Input: part model. Units: mm. Frame: model coordinates. Face numbers are marked on the shaded views. A direction names the side the tool comes from. Give positions to 0.01 mm unless a question says otherwise; leave off trailing zeros. Write each loop counter-clockwise with the first axis right and the second up, starting at its lowest first coordinate (ties: lowest second). Pieces come first, ordered by that corner, then holes.
```python
from build123d import *

# Parameters (mm, degrees)
F0_W     = 200
F0_H     = 50
F1_DEPTH = 40
F2_W     = 38
F2_H     = 28
F3_DEPTH = 200.001
F4_R     = 1
F5_DEPTH = 8
F6_R     = 1
F7_DEPTH = 8


with BuildPart() as f1:
    # F0 (on Top) → F1 (new body)
    with BuildSketch(Plane.XY):
        with Locations((40.836534, -29.115389)):
            Rectangle(F0_W, F0_H)
    extrude(amount=F1_DEPTH)

    # F2 (on face) → F3 (cut, through all)
    with BuildSketch(Plane(origin=(-59.163466, 0, 0), x_dir=(0, -1, 0), z_dir=(-1, 0, 0))):
        with Locations((29.115389, 20)):
            Rectangle(F2_W, F2_H)
    extrude(amount=-F3_DEPTH, mode=Mode.SUBTRACT)

    # F4 (on face) → F5 (cut)
    with BuildSketch(Plane(origin=(-59.163466, 0, 0), x_dir=(0, -1, 0), z_dir=(-1, 0, 0))):
        with Locations((8.115389, 36)):
            Circle(F4_R)
        with Locations((8.115389, 4)):
            Circle(F4_R)
        with Locations((50.115389, 4)):
            Circle(F4_R)
        with Locations((50.115389, 36)):
            Circle(F4_R)
    extrude(amount=-F5_DEPTH, mode=Mode.SUBTRACT)

    # F6 (on face) → F7 (cut)
    with BuildSketch(Plane.YZ.offset(140.836534)):
        with Locations((-50.115389, 36)):
            Circle(F6_R)
        with Locations((-8.115389, 36)):
            Circle(F6_R)
        with Locations((-8.115389, 4)):
            Circle(F6_R)
        with Locations((-50.115389, 4)):
            Circle(F6_R)
    extrude(amount=-F7_DEPTH, mode=Mode.SUBTRACT)


solid = f1.part
```
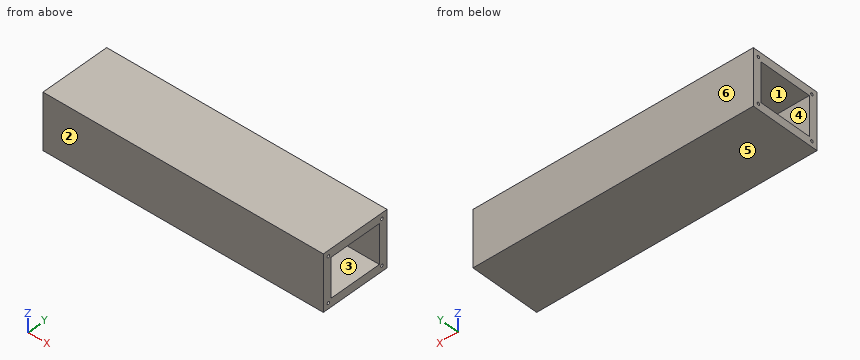
Item 1: Mould query, pull axis Y, two halves, no side actions, for the marked faces 3, 4, 5 and 6. Classes: +Y half, -Y half, draft (parallel to the pull), parting line (faces both ways), or undercut.
Item 2: Set-up query: the marked faces 1 and 2. Return all of +Z, -Z, +X, -X, +Y, -Y with unobstructed straight access to the full face (end or side cutting, diameter ignored); none if empty.
Item 3: Section C-C (y = -14). Return loops of the section in (x, z), and give its area (3 significant figures).
Item 4: Ray query, line 1 (Y direction, x = 104.5, z = 30.5); line 2 (Z direction, x = -46.5, y = -14.5). Return the intervals inside material, ascending.
Item 5: Section B-B (z = 10.5). Return loops of the section in (x, y).
Item 6: Section A-A (x = 84). Return loops of the section in (y, z), and give its area (3 significant figures).
Item 7: Pin query (flat end, axial travel): pin 1 (1 mm diameter, centred on x = 27.5, y = -41, fed in from -Z); pin 2 (0.6 mm diameter, centred on y = -49.5, z = 4, fed in from +X); pin 3 (1.8 mm diameter, centred on y = -8.12, z = 36, fed in from -X). Return the tip coordinate at first contact, or that it passes through.
Solved:
1. face 3: undercut
1. face 4: undercut
1. face 5: draft
1. face 6: +Y half
2. face 1: +X, -X
2. face 2: +Z, -Z, +X, -X, -Y
3. outline: (-59.16, 0) - (140.84, 0) - (140.84, 6) - (-59.16, 6) - close; (-59.16, 34) - (140.84, 34) - (140.84, 40) - (-59.16, 40) - close
3. area: 2,400 mm2
4. line 1: y = -54.12 to -48.12, -10.12 to -4.12
4. line 2: z = 0 to 6, 34 to 40
5. outline: (-59.16, -54.12) - (140.84, -54.12) - (140.84, -48.12) - (-59.16, -48.12) - close; (-59.16, -10.12) - (140.84, -10.12) - (140.84, -4.12) - (-59.16, -4.12) - close
6. outline: (-54.12, 0) - (-4.12, 0) - (-4.12, 40) - (-54.12, 40) - close; hole (-48.12, 6) - (-10.12, 6) - (-10.12, 34) - (-48.12, 34) - close
6. area: 936 mm2
7. pin 1: stops at z = 0
7. pin 2: stops at x = 132.84
7. pin 3: stops at x = -51.16
